```python
from build123d import *

# Parameters (mm, degrees)
BOX_W             = 5
BOX_H             = 6
BOX_DEPTH         = 8
CYLINDER001_R     = 1.675
CYLINDER001_DEPTH = 8
TORUS_R           = 2
CYLINDER_R        = 9
CYLINDER_DEPTH    = 14


with BuildPart() as d:
    # Box → Box (new body)
    with BuildSketch(Plane(origin=(1, -3, 15), x_dir=(1, 0, 0), z_dir=(0, 0, 1))):
        with Locations((2.5, 3)):
            Rectangle(BOX_W, BOX_H)
    extrude(amount=BOX_DEPTH)


with BuildPart() as eje_d:
    # Cylinder001 → Cylinder001 (new body)
    with BuildSketch(Plane.XY.offset(15)):
        Circle(CYLINDER001_R)
    extrude(amount=CYLINDER001_DEPTH)

    # Cut: cut D
    add(d.part, mode=Mode.SUBTRACT)


with BuildPart() as eje_d_1:
    # Cut placement: moved
    add(eje_d.part.moved(Location((0, 0, -9))))


with BuildPart() as obj1:
    # Torus → Torus (revolve)
    with BuildSketch(Plane(origin=(0, 0, 7), x_dir=(1, 0, 0), z_dir=(0, -1, 0))):
        with Locations((9, 0)):
            Circle(TORUS_R)
    revolve(axis=Axis((0, 0, 7), (0, 0, 1)))


with BuildPart() as obj2:
    # Cylinder → Cylinder (new body)
    with BuildSketch(Plane.XY):
        Circle(CYLINDER_R)
    extrude(amount=CYLINDER_DEPTH)

    # Cut001: cut obj1
    add(obj1.part, mode=Mode.SUBTRACT)

    # Cut002: cut EJE + D
    add(eje_d_1.part, mode=Mode.SUBTRACT)


solid = obj2.part
```
Verification items for the finished model (mm, model axes). A direction names the side the tool comes from. Coordinates: 2 decimals unless noted, no trailing zeros. Loops run counter-clockwise (first coordinate to the right, second up) from the corner with the lowest first, then second, coordinate; pieces in that order, holes last. Notation, with made-up numbers: (71, 26.25) - (128, 26.25) arc R23 ccw to (128, 37.25) - close; hole circle Ø3 at (23.25, 69). An arc over 180 degrees is marked (long way). Return JSON: item names as keys, results as strings.
1. Thickness scan on L1, parallel to Y at x = 0, z = 9.5 (3 decimals); L2, parallel to Z at x = 5.5, y = -5.75; L3, parallel to Z at x = -3.5, y = -7.5. Record the ranges inside material, lowest first.
Established:
{"L1": "y = -9 to -1.675, 1.675 to 9", "L2": "z = 0 to 5.29, 8.71 to 14", "L3": "z = 0 to 5.14, 8.86 to 14"}
2. Section check C-C, the plane z = 12.5. Record the boundary of the cut face in (x, y) (3 decimals), then the cut area to 3 significant figures.
Established:
{"outline": "circle Ø18 at (0, 0); hole (1, -1.344) - (1, 1.344) arc R1.675 ccw (long way) to start", "area": "247 mm2"}
3. Section check A-A, the plane x = 0. Record the boundary of the cut face in (y, z) (3 decimals), then the cut area to 3 significant figures.
Established:
{"outline": "(-9, 0) - (9, 0) - (9, 5) arc R2 cw to (9, 9) - (9, 14) - (1.675, 14) - (1.675, 6) - (-1.675, 6) - (-1.675, 14) - (-9, 14) - (-9, 9) arc R2 cw to (-9, 5) - close", "area": "213 mm2"}
4. Go/stop test with flat-tipped pins: pin 1 (1.5 mm diameter, centred on x = 2.5, z = 7, fed in from -Y); pin 2 (6 mm diameter, centred on y = -3.5, z = 2, fed in from +X); pin 3 (4 mm diameter, centred on x = -4.5, z = 11.5, fed in from +Y). Record where each tip stops, or that it passes through.
Established:
{"pin 1": "stops at y = -6.79", "pin 2": "stops at x = 8.99", "pin 3": "stops at y = 8.65"}
5. Section check B-B, the plane y = 0. Record the boundary of the cut face in (x, z) (3 decimals).
Established:
{"outline": "(-9, 0) - (9, 0) - (9, 5) arc R2 cw to (9, 9) - (9, 14) - (1, 14) - (1, 6) - (-1.675, 6) - (-1.675, 14) - (-9, 14) - (-9, 9) arc R2 cw to (-9, 5) - close"}
6. Mould release check, pull along X, two halves, no side actions. Record for faces 1 (the cylindrical face through (-1.172, 8.923, 11.465)), 2 (the flat face through (0, -2, 14)), 3 (the flat face through (1, 0, 10)): +X half, -X half, draft (parallel to the pull), parting line (faces both ways), or undercut.
Established:
{"face 1": "parting line", "face 2": "draft", "face 3": "undercut"}
7. Tool access check on faces 4 (the cylindrical face through (-1.172, 8.923, 2.465)), 5 (the cylindrical face through (-1.674, 0.052, 9.944)). Record the directions out of +Z, -Z, +X, -X, +Y, -Y that give a thin tool (end or side, any length) a straight path to the whole face; none if there is none.
Established:
{"face 4": "+Z, -Z", "face 5": "+Z"}
8. Section check D-D, the plane z = 3.75. Record the boundary of the cut face in (x, y), then the cut area to 3 significant figures.
Established:
{"outline": "circle Ø18 at (0, 0)", "area": "254 mm2"}
